Source: CAD feature listing. Evaluate the final solid. Frame: model axes, mm. Face numbers are marked on the shaded views. A direction names the side the tool comes from. Give positions to 0.01 mm unless a question says otherwise; leave off trailing zeros. Loops run counter-clockwise (first coordinate to the right, second up) from the corner with the lowest first, then second, coordinate; pieces in that order, holes last. Notation, with made-up numbers: (14.25, -17.75) - (21.25, -17.75) arc R6 ccw to (21.25, -13.75) - close; hole circle Ø5 at (38, -32.5). An arc over 180 degrees is marked (long way). Put each result on its own line as item: value.
```python
from build123d import *

# Parameters (mm, degrees)
ESBO_O1_R                = 1.25
RESSALTO_EXTRUS_O1_DEPTH = 2
ESBO_O3_W                = 10
ESBO_O3_H                = 3
RESSALTO_EXTRUS_O2_DEPTH = 7
ESBO_O4_R                = 1.75
CORTE_EXTRUS_O1_DEPTH    = 5


with BuildPart() as part:
    # Esbo_o1 → Ressalto-extrus_o1 (new body)
    with BuildSketch(Plane.XY):
        Polygon((-13.965681545, 17.117604611), (-13.965681545, -11.882395389), (-9.965681545, -11.882395389), (-9.965681545, -7.382395389), (38.034318455, -7.382395389), (38.034318455, -11.882395389), (42.034318455, -11.882395389), (42.034318455, 17.117604611), (38.034318455, 17.117604611), (38.034318455, 12.617604611), (-9.965681545, 12.617604611), (-9.965681545, 17.117604611), align=None)
        with Locations((-11.365681545, 14.367604611)):
            Circle(ESBO_O1_R, mode=Mode.SUBTRACT)
        with Locations((-11.365681545, -9.132395389)):
            Circle(ESBO_O1_R, mode=Mode.SUBTRACT)
        with Locations((39.434318455, -9.132395389)):
            Circle(ESBO_O1_R, mode=Mode.SUBTRACT)
        with Locations((39.434318455, 14.367604611)):
            Circle(ESBO_O1_R, mode=Mode.SUBTRACT)
    extrude(amount=RESSALTO_EXTRUS_O1_DEPTH)

    # Esbo_o3 → Ressalto-extrus_o2 (add)
    with BuildSketch(Plane.XY.offset(2)):
        with Locations((-8.965681545, -13.382395389)):
            Rectangle(ESBO_O3_W, ESBO_O3_H)
        with Locations((37.034318455, -13.382395389)):
            Rectangle(ESBO_O3_W, ESBO_O3_H)
    extrude(amount=-RESSALTO_EXTRUS_O2_DEPTH)

    # Esbo_o4 → Corte-extrus_o1 (cut)
    with BuildSketch(Plane(origin=(0, -11.882395389, 0), x_dir=(1, 0, 0), z_dir=(0, 1, 0))):
        with Locations((-11.465681545, 2.5)):
            Circle(ESBO_O4_R)
        with Locations((39.534318455, 2.5)):
            Circle(ESBO_O4_R)
    extrude(amount=-CORTE_EXTRUS_O1_DEPTH, mode=Mode.SUBTRACT)


solid = part.part
```
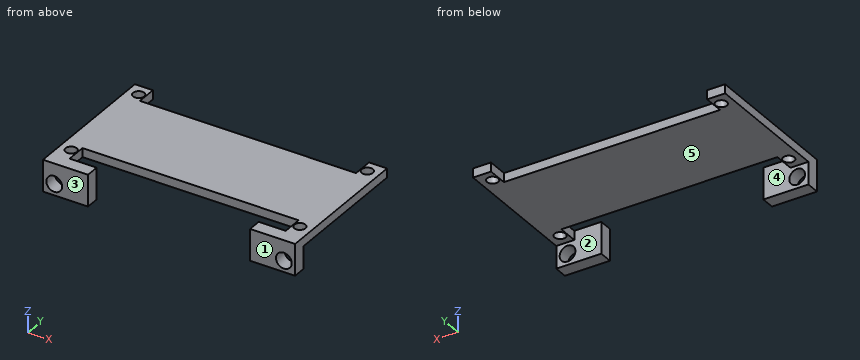
1) Section query B-B, the plane y = 7. Output: boundary loops of the cut face in (x, z), plus the area to 3 significant figures.
Check result:
outline: (-13.97, 0) - (42.03, 0) - (42.03, 2) - (-13.97, 2) - close
area: 112 mm²
2) Section query D-D, the plane x = 29. Output: boundary loops of the cut face in (y, z), plus the area to 3 significant figures.
Check result:
outline: (-7.38, 0) - (12.62, 0) - (12.62, 2) - (-7.38, 2) - close
area: 40.0 mm²
3) Material intervals for line 1 along X through (y, z) = (-9, 0.5); line 2 along Y through (x, z) = (26, 0.5); line 3 along Z through (x, y) = (21, 2.5), sorted ascending. Write a range as [from, to].
Check result:
line 1: [-13.97, -12.61], [-10.12, -9.97], [38.03, 38.19], [40.68, 42.03]
line 2: [-7.38, 12.62]
line 3: [0, 2]
4) Pin query (flat end, axial travel): P1, Ø3, axis at x = 23, z = 0.5, coming from the +Y side; P2, Ø8, axis at x = 26.5, y = -11, coming from the -Z side; P3, Ø1, axis at x = 22, z = 1.5, coming from the -Y side. Return the tip coordinate at first contact, or that it passes through.
Check result:
P1: y = 12.62
P2: z = 0
P3: y = -7.38
5) Section query A-A, the plane z = -2.5. Output: boundary loops of the cut face in (x, y), plus the area to 3 significant figures.
Check result:
outline: (-13.97, -14.88) - (-13.22, -14.88) - (-13.22, -11.88) - (-13.97, -11.88) - close; (-9.72, -14.88) - (-3.97, -14.88) - (-3.97, -11.88) - (-9.72, -11.88) - close; (32.03, -14.88) - (37.78, -14.88) - (37.78, -11.88) - (32.03, -11.88) - close; (41.28, -14.88) - (42.03, -14.88) - (42.03, -11.88) - (41.28, -11.88) - close
area: 39.0 mm²
6) Access query for the marked faces 3, 4 and 5. Directions: +Z, -Z, +X, -X, +Y, -Y. A direction counts if a zero-diameter tool reaches every point of the face in a straight line with its end or side. Return the directions, or none.
Check result:
face 3: +Z, -Z, +X, -X, -Y
face 4: -Z
face 5: -Z, +X, -X, +Y
7) Section query C-C, the plane z = 0.75. Output: boundary loops of the cut face in (x, y), plus the area to 3 significant figures.
Check result:
outline: (-13.97, -14.88) - (-3.97, -14.88) - (-3.97, -11.88) - (-9.97, -11.88) - (-9.97, -7.38) - (38.03, -7.38) - (38.03, -11.88) - (32.03, -11.88) - (32.03, -14.88) - (42.03, -14.88) - (42.03, 17.12) - (38.03, 17.12) - (38.03, 12.62) - (-9.97, 12.62) - (-9.97, 17.12) - (-13.97, 17.12) - close; hole circle Ø2.5 at (-11.37, -9.13); hole circle Ø2.5 at (-11.37, 14.37); hole circle Ø2.5 at (39.43, -9.13); hole circle Ø2.5 at (39.43, 14.37)
area: 1,230 mm²
8) Mould query, pull axis X, two halves, no side actions, for the marked faces 1 and 2. Classes: pulls with the +X half, pulls with the -X half, needs draft (parallel to the pull), parting line crosses it, or undercut.
Check result:
face 1: needs draft
face 2: undercut
